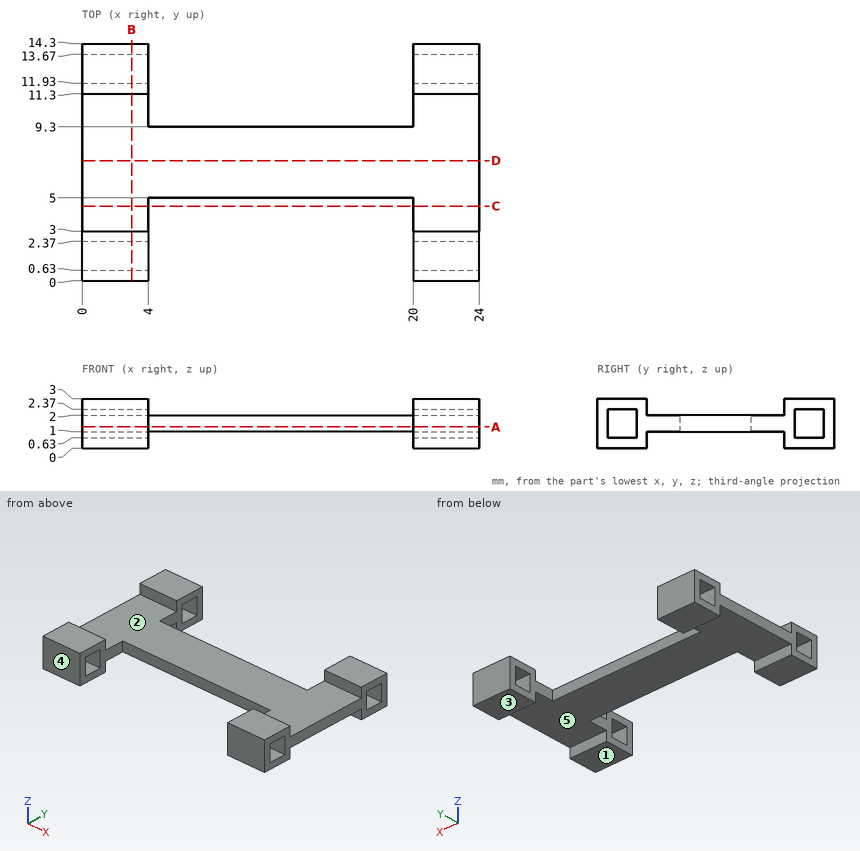
Design review of the part shown in the three views and the two pictorial views. Dimensions are in mm from the part's minimum x, y and z. A direction names the side the tool comes from. Round coordinates to 2 decimals unless told otherwise and drop trailing zeros. Write each loop counter-clockwise with the first axis right and the second up, starting at its lowest first coordinate (ties: lowest second). Pieces come first, ordered by that corner, then holes. Notation, with made-up numbers: (62.25, -37) -> (102.25, -37) arc R6 cw to (102.25, -27) -> close; hole circle Ø6 at (-24, -17.75). An arc over 180 degrees is marked (long way). One line per question, with ' | ' between items. Start each with the question number.
1) Wall thickness on line 1 along X through (y, z) = (11.5, 1.55); line 2 along Y through (x, z) = (22, 2.6); line 3 along Z through (x, y) = (21.25, 0.75): over which ranges is each line inside the solid? List them lowest first.
2) Mouldability with a two-part tool opening along Y and no side actions: class the marked faces 3, 4 and 5 as +Y half, -Y half, draft (parallel to the pull), parting line (faces both ways), or undercut.
3) Machinability: for the marked faces 1 and 2, which of the approach directions +Z, -Z, +X, -X, +Y, -Y give a long, thin tool a straight path to every point of the face, cutting with its end or side? Answer none if there is none.
4) Add section D-D (y = 7.25). Write out the cut boundary in (x, z), and give its area (3 significant figures).
5) For pin 1 Ø3 at (x, y) = (12.5, 5) entering from -Z; pin 2 Ø1.5 at (x, z) = (13, 1.5) entering from -Y, all flat-tipped, find the tip position at first contact; note any pin that passes through.
6) Add section A-A (z = 1.3). Write out the cut boundary in (x, y).
7) Add section B-B (x = 3). Write out the cut boundary in (y, z).
8) Add section C-C (y = 4.5). Write out the cut boundary in (x, z), and give its area (3 significant figures).
Reported:
1) line 1: x = 0 to 4, 20 to 24 | line 2: y = 0 to 3, 11.3 to 14.3 | line 3: z = 0 to 0.63, 2.37 to 3
2) face 3: draft | face 4: -Y half | face 5: undercut
3) face 1: -Z, +X, -X, +Y, -Y | face 2: +Z, +X, -X
4) outline: (0, 1) -> (24, 1) -> (24, 2) -> (0, 2) -> close | area: 24.0 mm²
5) pin 1: stops at z = 1 | pin 2: stops at y = 5
6) outline: (0, 0) -> (4, 0) -> (4, 0.63) -> (0, 0.63) -> close; (0, 2.37) -> (4, 2.37) -> (4, 5) -> (20, 5) -> (20, 2.37) -> (24, 2.37) -> (24, 11.93) -> (20, 11.93) -> (20, 9.3) -> (4, 9.3) -> (4, 11.93) -> (0, 11.93) -> close; (0, 13.67) -> (4, 13.67) -> (4, 14.3) -> (0, 14.3) -> close; (20, 0) -> (24, 0) -> (24, 0.63) -> (20, 0.63) -> close; (20, 13.67) -> (24, 13.67) -> (24, 14.3) -> (20, 14.3) -> close
7) outline: (0, 0) -> (3, 0) -> (3, 1) -> (11.3, 1) -> (11.3, 0) -> (14.3, 0) -> (14.3, 3) -> (11.3, 3) -> (11.3, 2) -> (3, 2) -> (3, 3) -> (0, 3) -> close; hole (0.63, 0.63) -> (2.37, 0.63) -> (2.37, 2.37) -> (0.63, 2.37) -> close; hole (11.93, 0.63) -> (13.67, 0.63) -> (13.67, 2.37) -> (11.93, 2.37) -> close
8) outline: (0, 1) -> (4, 1) -> (4, 2) -> (0, 2) -> close; (20, 1) -> (24, 1) -> (24, 2) -> (20, 2) -> close | area: 8.00 mm²
